Autodesk Inventor part; units mm, degrees
ref_plane "YZ Plane" through (0, 0, 0) normal (1, 0, 0) x (0, 1, 0)
ref_plane "XZ Plane" through (0, 0, 0) normal (0, 1, 0) x (-1, 0, 0)
ref_plane "XY Plane" through (0, 0, 0) normal (0, 0, 1) x (1, 0, 0)
sketch "スケッチ1" plane through (0, 0, 0) normal (0, 1, 0) x (-1, 0, 0)
  arc A0 (99.4141, -32.927) -> (197.8245, -22.9934) centre (88.5018, 567.6156) ccw
  arc A1 (73.8469, -32.6347) -> (99.4141, -32.927) centre (91.566, 398.982) ccw
  arc A2 (27.3573, -24.3709) -> (73.8469, -32.6347) centre (81.048, 142.776) ccw
  arc A3 (0.844, -11.3484) -> (27.3573, -24.3709) centre (58.458, 72.45) ccw
  arc A4 (-6.1834, -4.5246) -> (0.844, -11.3484) centre (17.4, 12.732) ccw
  arc A5 (-1.3535, 7.5415) -> (-6.1834, -4.5246) centre (0, 0) ccw
  arc A6 (18.2937, 9.3227) -> (-1.3535, 7.5415) centre (18.66, -103.968) ccw
  arc A7 (38.1205, 9.1058) -> (18.2937, 9.3227) centre (20.556, -690.396) ccw
  arc A8 (197.8245, -22.9934) -> (38.1205, 9.1058) centre (-36.3979, -774.9853) ccw
  circle A9 centre (20, -2.2582) radius 6
  circle A10 centre (130, -14.678) radius 6
extrude "押し出し2" add sketch "スケッチ1" along normal mid plane 44.75
properties part number "uretan_mc" material "ポリエチレン、高密度"
Source: CAD feature listing. Evaluate the final solid. Frame: model axes, mm. Coordinates: 2 decimals unless noted, no trailing zeros. Loops run counter-clockwise (first coordinate to the right, second up) from the corner with the lowest first, then second, coordinate; pieces in that order, holes last. Notation, with made-up numbers: (24.25, 48.5) - (30.25, 48.5) arc R21 cw to (30.25, 83.5) - close; hole circle Ø11 at (31, 4). An arc over 180 degrees is marked (long way). One line per question, with ' | ' between items.
1) Section B-B, the plane z = -17. Return loops of the section in (x, y) (3 decimals).
Report:
outline: (-177.635, -22.375) - (-135.532, -22.375) - (-135.532, 22.375) - (-177.635, 22.375) - close; (-124.468, -22.375) - (-10.082, -22.375) - (-10.082, 22.375) - (-124.468, 22.375) - close
2) Line query: line 1 along Z through (x, y) = (-130, 8.5); line 2 along Z through (x, y) = (-20, 12.5); line 3 along Z through (x, y) = (-43, 10). Output: solid intervals per line, ascending.
Report:
line 1: z = -31.59 to -20.68, -8.68 to -5.14 | line 2: z = -21.69 to -8.26, 3.74 to 9.33 | line 3: z = -28.61 to 8.63
3) Section C-C, the plane y = 11. Return loops of the section in (x, z), then the cut area to 4 significant figures.
Report:
outline: (-197.82, -22.99) arc R600.64 ccw to (-99.41, -32.93) arc R432.03 ccw to (-73.85, -32.63) arc R175.56 ccw to (-27.36, -24.37) arc R101.69 ccw to (-0.84, -11.35) arc R29.22 ccw to (6.18, -4.52) arc R7.66 ccw to (1.35, 7.54) arc R113.29 ccw to (-18.29, 9.32) arc R700.07 ccw to (-38.12, 9.11) arc R787.62 ccw to start; hole circle Ø12 at (-130, -14.68); hole circle Ø12 at (-20, -2.26) | area: 5,175 mm²
4) Pull-direction query (X, two-part tool) for faces 1 (the face through (-25.542, -0.313, 0.04)), 2 (the face through (-50.65, -0.31, -30.13)), 3 (the face through (-149.51, -0.31, -29.92)); classes: released by +X, released by -X, zero draft, split by the parting line, or undercut.
Report:
face 1: undercut | face 2: released by +X | face 3: released by -X
5) Section A-A, the plane x = -130. Return loops of the section in (y, z) (3 decimals).
Report:
outline: (-22.375, -31.591) - (22.375, -31.591) - (22.375, -20.678) - (-22.375, -20.678) - close; (-22.375, -8.678) - (22.375, -8.678) - (22.375, -5.139) - (-22.375, -5.139) - close
6) First-contact query: P1, Ø6, axis at x = -61, y = -13.5, coming from the -Z side; P2, Ø2, axis at x = -68.5, y = -0.5, coming from the -Z side; P3, Ø19, axis at x = -130, z = -14.678, coming from the -Y side (3 decimals); P4, Ø1.5, axis at x = -22, y = 14.5, coming from the -Z side. Flat tips, straight axial feed; report the tip coordinate or a pass-through.
Report:
P1: stops at z = -31.95 | P2: stops at z = -32.4 | P3: stops at y = -22.375 | P4: stops at z = -22.77
